CAD build for the part. Positions are in the model's coordinates, mm. A direction names the side the tool comes from. Round coordinates to 2 decimals unless told otherwise and drop trailing zeros. Loops run counter-clockwise (first coordinate to the right, second up) from the corner with the lowest first, then second, coordinate; pieces in that order, holes last. Notation, with made-up numbers: (42, 87.5) - (86, 87.5) arc R32 ccw to (86, 123.5) - close; hole circle Ø1 at (-35.5, 39.25). An arc over 180 degrees is marked (long way). Use one line per item in the form item = value.
Autodesk Inventor part; units mm, degrees
sketch "Эскиз1" plane through (0, 0, 0) normal (0, 1, 0) x (-1, 0, 0)
  circle A0 centre (0, 0) radius 11.2
  circle A1 centre (0, 0) radius 13.2
  circle A2 centre (0, 0) radius 5.5
  dimension "d0" = 22.4
  dimension "d1" = 2
  dimension "d2" = 11
extrude "Выдавливание1" add sketch "Эскиз1" along normal blind 22 contours A1
extrude "Выдавливание2" add sketch "Эскиз1" against normal blind 2 contours A0 | A1
fillet "Сопряжение1" radius 1 2 edges at (13.2, 22, 0) (11.2, 22, 0)
sketch "Эскиз2" plane through (0, 0, 0) normal (1, 0, 0) x (0, 1, 0)
  line L0 (-53, 0) -> (-53, -8)
  line L1 (-53, 0) -> (-2, 0)
  line L2 (-69.0693, 0) -> (-63.203, 0)
  line L3 (-2, 13.2) -> (-2, -13.2)
  line L4 (-2, 13.2) -> (-2, -13.2)
  line L5 (-53, -8) -> (-2, -13.2)
  point P0 (0, 0)
  dimension "d13" = 51
  dimension "d14" = 8
revolve "Вращение1" add sketch "Эскиз2" angle 360 about axis through (0, -69.0693, 0) along (0, 1, 0)
extrude "Выдавливание3" cut sketch "Эскиз1" against normal up to surface (53 mm away) contours A2
sketch "Эскиз5" plane through (0, -53, 0) normal (0, -1, 0) x (1, 0, 0)
  circle A0 centre (0, 0) radius 5.15
  circle A1 centre (0, 0) radius 5.5
  dimension "d18" = 10.3
extrude "Выдавливание4" add sketch "Эскиз5" against normal blind 46
properties part number "Стакан для крепления ходовой гайки"
1) Tool access for faces 1 (the cylindrical face through (11.19, 10.35, -0.49)), 2 (the conical face through (-10.546, -27.143, 1.385)): list every direction of +Z, -Z, +X, -X, +Y, -Y with a clear straight run to the whole face (end or side of a thin tool).
Report:
face_1 = +Y
face_2 = -Y
2) Drill centre lines: probe 1 along Z at (x, y) = (0, 11); probe 2 along Y at (x, z) = (-4.25, -6.75); probe 3 along Z at (x, y) = (-4.5, 3). Where is each one in solid material? Low to high.
Report:
probe_1 = -13.2 to -11.2, 11.2 to 13.2
probe_2 = -53 to 0
probe_3 = -12.41 to -10.26, 10.26 to 12.41
3) Slice it at D-D (y = -43.5). Write the cut outline in (x, z).
Report:
outline = circle Ø17.94 at (0, 0); hole circle Ø10.3 at (0, 0)
4) Flat gauge pins, fed straight in: pin 1 (6.5 mm diameter, centred on x = 1, z = 0, fed in from +Y); pin 2 (3 mm diameter, centred on x = 7.5, y = -25, fed in from -Z); pin 3 (1 mm diameter, centred on x = -6.5, y = 5.5, fed in from +Z); pin 4 (14.5 mm diameter, centred on x = 0, z = 0, fed in from +Y). Where does each tip first touch, or does it go through?
Report:
pin_1 = through
pin_2 = -9.06
pin_3 = 11.76
pin_4 = 0
5) Slice it at C-C (y = -18.5). Write the cut outline in (x, z).
Report:
outline = circle Ø23.04 at (0, 0); hole circle Ø10.3 at (0, 0)
6) Two-plate mould, pull along Z, no slides. Class faces 3 (the cylindrical face through (9.73, 9.34, -8.92)), 4 (the flat face through (5, -53, -2)), 5 (the cylindrical face through (4.91, -30.32, 1.55)): +Z half, -Z half, draft (parallel to the pull), parting line (faces both ways), or undercut.
Report:
face_3 = parting line
face_4 = draft
face_5 = undercut
